Check sheet for the modelled part. Datum: model origin and axes. Units: mm. Face numbers are marked on the shaded views. A direction names the side the tool comes from. Coordinates: 2 decimals unless noted, no trailing zeros. Loops run counter-clockwise (first coordinate to the right, second up) from the corner with the lowest first, then second, coordinate; pieces in that order, holes last. Notation, with made-up numbers: (-23, -21) - (-8, -21) arc R27 cw to (-8, 11) - close; hole circle Ø4 at (2.5, 13.5). An arc over 180 degrees is marked (long way). Write each question's results on one line, items separated by ' | '. Start each with the question number.
1. Draft check along X on the marked faces 1, 2 and 3. Enter one of: released by +X, released by -X, zero draft, split by the parting line, or undercut.
2. Cross-section at A-A (z = -22.5). Record the cut outline in (x, y), and give its area (3 significant figures).
3. Cross-section at C-C (x = 22.5). Record the cut outline in (y, z).
4. Thickness scan on line 1 (Z direction, x = 22.5, y = 10.1); line 2 (X direction, y = 6.75, z = -21); line 3 (X direction, y = 6.5, z = -18). Record the ranges inside material, lowest first. Write a range as [from, to].
5. Gauge pin test, flat ends, axial feed: P1, Ø1.5, axis at x = 19, z = -35.5, coming from the +Y side; P2, Ø1.5, axis at x = 5, y = 6.5, coming from the +Z side; P3, Ø3, axis at x = 8, y = 8, coming from the -Z side. Record the tip position at first contact, or that the pin passes through.
6. Cross-section at B-B (y = 14.25). Record the cut outline in (x, z), and give its area (3 significant figures).
7. Tool access check on the marked faces 4, 5, 6, 7 and 8. Record the directions out of +Z, -Z, +X, -X, +Y, -Y that give a thin tool (end or side, any length) a straight path to the whole face; none if there is none.
8. Cross-section at D-D (x = 37). Record the cut outline in (y, z), and give its area (3 significant figures).
```python
from build123d import *

# Parameters (mm, degrees)
SKETCH_1_W               = 45
SKETCH_1_H               = 45
EXTRUDE_1_DEPTH          = 16
CUT_EXTRUDE_1_DEPTH      = 66.620118866
SKETCH_3_W               = 13.364101615
SKETCH_3_H               = 45
CUT_EXTRUDE_2_DEPTH      = 8
CUT_EXTRUDE_3_REACH      = 67.62
FILLET_1_R               = 6
F_2MM_W                  = 50.544050544
F_2MM_H                  = 52.749609113
CUT_EXTRUDE_4_DEPTH      = 2
EXTRUDE_2_DEPTH          = 6
SKETCH_6_R               = 2.5
CUT_EXTRUDE_5_DEPTH      = 30
EXTRUDE_3_DEPTH          = 2
SKETCH_9_W               = 20
SKETCH_9_H               = 10
EXTRUDE_4_DEPTH          = 8
FILLET_2_R               = 5
CUT_EXTRUDE_6_DEPTH      = 5
FILLET_3_R               = 3
HOLE_WIZARD_M41_D        = 4.5
M4X0_71_D                = 3.3
CUT_EXTRUDE_7_REACH      = 73.631
CUT_EXTRUDE_7_END_RADIUS = 2.5
M4X0_72_D                = 3.3


with BuildPart() as part:
    # Эскиз1 → Бобышка-Вытянуть1 (new body)
    with BuildSketch(Plane(origin=(0, 0, 0), x_dir=(1, 0, 0), z_dir=(0, 1, 0))):
        with Locations((22.5, 22.5)):
            Rectangle(SKETCH_1_W, SKETCH_1_H)
    extrude(amount=EXTRUDE_1_DEPTH)

    # Эскиз2 → Вырез-Вытянуть1 (cut, through all)
    with BuildSketch(Plane.XY):
        Polygon((8.745299462, 8), (36.254700538, 8), (31.635898385, 0), (13.364101615, 0), align=None)
    extrude(amount=-CUT_EXTRUDE_1_DEPTH, mode=Mode.SUBTRACT)

    # Эскиз3 → Вырез-Вытянуть2 (cut)
    with BuildSketch(Plane.XZ):
        with Locations((38.317949193, -22.5)):
            Rectangle(SKETCH_3_W, SKETCH_3_H)
    extrude(amount=-CUT_EXTRUDE_2_DEPTH, mode=Mode.SUBTRACT)

    # Эскиз4 → Вырез-Вытянуть3 (cut, up to next)
    with BuildSketch(Plane(origin=(45, 0, 0), x_dir=(0, 0, -1), z_dir=(1, 0, 0)), mode=Mode.PRIVATE) as cut_extrude_3_sk1:
        Polygon((5.082050808, 16), (2.195299462, 11), (42.804700538, 11), (39.917949192, 16), align=None)
    cut_extrude_3_tool1 = extrude(cut_extrude_3_sk1.sketch, amount=-CUT_EXTRUDE_3_REACH, mode=Mode.PRIVATE) & part.part
    add(cut_extrude_3_tool1.solids().sort_by_distance((45, 13.436229, -22.5))[0], mode=Mode.SUBTRACT)

    # Скругление1
    fillet_1_edges = [part.edges().sort_by_distance(p)[0] for p in [
        (0, 8, -45),
        (45, 12, -45),
        (45, 12, 0),
        (0, 8, 0),
    ]]
    fillet(fillet_1_edges, radius=FILLET_1_R)

    # -2mm → Вырез-Вытянуть4 (cut)
    with BuildSketch(Plane.XZ):
        with Locations((21.76481381, -22.637847411)):
            Rectangle(F_2MM_W, F_2MM_H)
    extrude(amount=-CUT_EXTRUDE_4_DEPTH, mode=Mode.SUBTRACT)

    # Эскиз7 → Бобышка-Вытянуть2 (add)
    with BuildSketch(Plane.XZ.offset(-8)):
        with BuildLine():
            Line((43, -39), (43, -6))
            ThreePointArc((43, -6), (41.828427125, -3.171572875), (39, -2))
            Line((39, -2), (36, -2))
            Line((36, -2), (36, 0))
            Line((36, 0), (39, 0))
            ThreePointArc((39, 0), (43.242640687, -1.757359313), (45, -6))
            Line((45, -6), (45, -39))
            ThreePointArc((45, -39), (43.242640687, -43.242640687), (39, -45))
            Line((39, -45), (36, -45))
            Line((36, -45), (36, -43))
            Line((36, -43), (39, -43))
            ThreePointArc((39, -43), (41.828427125, -41.828427125), (43, -39))
        make_face()
    extrude(amount=EXTRUDE_2_DEPTH)

    # Эскиз6 → Вырез-Вытянуть5 (cut)
    with BuildSketch(Plane.XY):
        with Locations((4.352411604, 6.5)):
            Circle(SKETCH_6_R)
    extrude(amount=-CUT_EXTRUDE_5_DEPTH, mode=Mode.SUBTRACT)

    # Эскиз8 → Бобышка-Вытянуть3 (add)
    with BuildSketch(Plane.XZ.offset(-8)):
        with BuildLine():
            Line((36, -2), (39, -2))
            ThreePointArc((39, -2), (41.828427125, -3.171572875), (43, -6))
            Line((43, -6), (43, -39))
            ThreePointArc((43, -39), (41.828427125, -41.828427125), (39, -43))
            Line((39, -43), (36, -43))
            Line((36, -43), (36, -2))
        make_face()
    extrude(amount=EXTRUDE_3_DEPTH)

    # Эскиз9 → Бобышка-Вытянуть4 (add)
    with BuildSketch(Plane(origin=(0, 16, 0), x_dir=(1, 0, 0), z_dir=(0, 1, 0))):
        with Locations((22.5, 50)):
            Rectangle(SKETCH_9_W, SKETCH_9_H)
    extrude(amount=-EXTRUDE_4_DEPTH)

    # Скругление2
    fillet_2_edges = [part.edges().sort_by_distance(p)[0] for p in [
        (32.5, 12, -55),
        (12.5, 12, -55),
    ]]
    fillet(fillet_2_edges, radius=FILLET_2_R)

    # Эскиз10 → Вырез-Вытянуть6 (cut)
    with BuildSketch(Plane(origin=(0, 16, 0), x_dir=(1, 0, 0), z_dir=(0, 1, 0))):
        with BuildLine():
            Line((14.5, 50), (14.5, 39.917949192))
            Line((14.5, 39.917949192), (30.5, 39.917949192))
            Line((30.5, 39.917949192), (30.5, 50))
            ThreePointArc((30.5, 50), (29.621320344, 52.121320344), (27.5, 53))
            Line((27.5, 53), (17.5, 53))
            ThreePointArc((17.5, 53), (15.378679656, 52.121320344), (14.5, 50))
        make_face()
    extrude(amount=-CUT_EXTRUDE_6_DEPTH, mode=Mode.SUBTRACT)

    # Скругление3
    fillet_3_edges = [part.edges().sort_by_distance(p)[0] for p in [
        (32.5, 12, -45),
        (12.5, 12, -45),
    ]]
    fillet(fillet_3_edges, radius=FILLET_3_R)

    # Отверстие с зазором M41 (through all)
    with Locations(Plane(origin=(0, 11, 0), x_dir=(1, 0, 0), z_dir=(0, 1, 0))):
        with Locations((22.5, 47.902350269)):
            Hole(HOLE_WIZARD_M41_D / 2)

    # Отверстие обработанное метчиком M4x0.71 (through all)
    with Locations(Plane(origin=(0, 6, 0), x_dir=(-1, 0, 0), z_dir=(0, -1, 0))):
        with Locations((-39.5, 22.5)):
            Hole(M4X0_71_D / 2)

    # Вырез-Вытянуть7: up to this cylinder (the profile starts outside it)
    cut_extrude_7_end = Plane(origin=(4.352411604, 6.5, -14.25), z_dir=(0, 0, 1)) * Cylinder(CUT_EXTRUDE_7_END_RADIUS, 153.262, mode=Mode.PRIVATE)
    # Эскиз17 → Вырез-Вытянуть7 (cut, up to the surface)
    with BuildSketch(Plane(origin=(0, 11, 0), x_dir=(1, 0, 0), z_dir=(0, 1, 0)), mode=Mode.PRIVATE) as cut_extrude_7_sk1:
        with BuildLine():
            Line((6.102411604, 17.5), (6.102411604, 11))
            ThreePointArc((6.102411604, 11), (4.352411604, 9.25), (2.602411604, 11))
            Line((2.602411604, 11), (2.602411604, 17.5))
            ThreePointArc((2.602411604, 17.5), (4.352411604, 19.25), (6.102411604, 17.5))
        make_face()
    cut_extrude_7_tool1 = extrude(cut_extrude_7_sk1.sketch, amount=-CUT_EXTRUDE_7_REACH, mode=Mode.PRIVATE) - cut_extrude_7_end
    add(cut_extrude_7_tool1.solids().sort_by_distance((4.352412, 11, -14.25))[0], mode=Mode.SUBTRACT)

    # Отверстие обработанное метчиком M4x0.72 (through all)
    with Locations(Plane(origin=(0, 8, 0), x_dir=(-1, 0, 0), z_dir=(0, -1, 0))):
        with Locations((-22.372649731, 22.5)):
            Hole(M4X0_72_D / 2)


solid = part.part
```
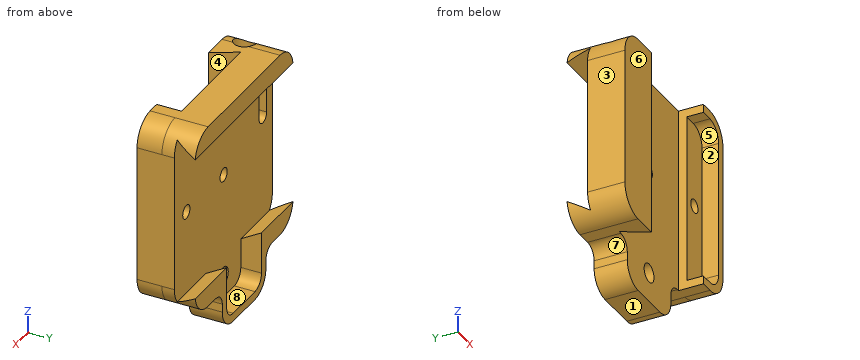
Established:
1) face 1: zero draft | face 2: undercut | face 3: released by -X
2) outline: (0, 2) - (12.21, 2) - (8.75, 8) - (20.72, 8) - (20.72, 11) - (0, 11) - close; (24.02, 8) - (36, 8) - (36, 6) - (37.85, 6) - (37.85, 11) - (24.02, 11) - close; (41.15, 6) - (43, 6) - (43, 2) - (45, 2) - (45, 11) - (41.15, 11) - close; hole circle Ø5 at (4.35, 6.5) | area: 178 mm^2
3) outline: (8, -55) - (16, -55) - (16, -53) - (11, -53) - (11, -50.15) - (8, -50.15) - close; (8, -45.65) - (11, -45.65) - (11, -24.15) - (8, -24.15) - close; (8, -20.85) - (11, -20.85) - (11, -2.2) - (16, -5.08) - (16, 0) - (8, 0) - close
4) line 1: [-55, -50.15], [-45.65, -24.15], [-20.85, 0] | line 2: [0, 1.86], [6.84, 9.47], [36, 38.81], [40.19, 45] | line 3: [0, 1.85], [6.85, 9.61], [36, 45]
5) P1: y = 11 | P2: z = -30 | P3: z = -45
6) outline: (0.32, -40.93) arc R6 ccw to (6, -45) - (9.5, -45) arc R3 cw to (12.5, -48) - (12.5, -50) arc R5 ccw to (17.5, -55) - (27.5, -55) arc R5 ccw to (32.5, -50) - (32.5, -48) arc R3 cw to (35.5, -45) - (39, -45) arc R6 ccw to (44.68, -40.93) - (30.5, -40.93) - (30.5, -50) arc R3 cw to (27.5, -53) - (17.5, -53) arc R3 cw to (14.5, -50) - (14.5, -40.93) - close; (0.32, -4.07) - (44.68, -4.07) arc R6 ccw to (39, 0) - (6, 0) arc R6 ccw to start | area: 340 mm^2
7) face 4: +Z, -Z | face 5: -Y | face 6: +Z, -Z, +X, -X, -Y | face 7: -Z, -X, +Y, -Y | face 8: +Y
8) outline: (2, -45) - (16, -45) - (16, -39.92) - (11, -42.8) - (11, -2.2) - (16, -5.08) - (16, 0) - (2, 0) - (2, -2) - (6, -2) - (6, -43) - (2, -43) - close | area: 277 mm^2
